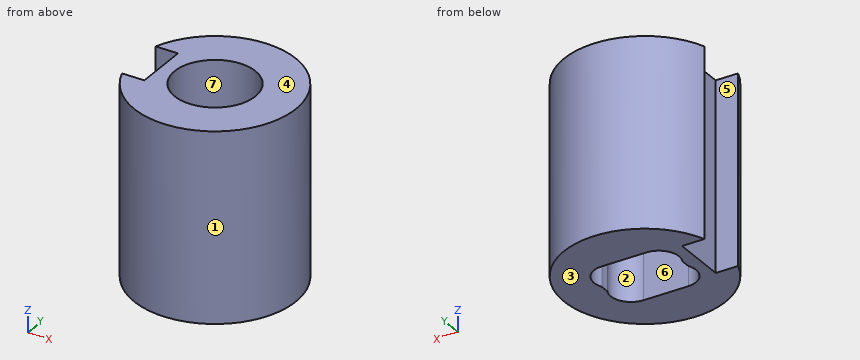
```python
from build123d import *

# Parameters (mm, degrees)
EXTRUDE_1_DEPTH     = 28
CUT_EXTRUDE_1_DEPTH = 10
SKETCH_3_R          = 6
CUT_EXTRUDE_2_DEPTH = 18


with BuildPart() as part:
    # Эскиз1 → Бобышка-Вытянуть1 (new body)
    with BuildSketch(Plane(origin=(0, 0, -1), x_dir=(-1, 0, 0), z_dir=(0, 0, -1))):
        with BuildLine():
            Line((11.313708499, 4), (8, 4))
            Line((8, 4), (8, -4))
            Line((8, -4), (11.313708499, -4))
            ThreePointArc((11.313708499, -4), (-12, 0), (11.313708499, 4))
        make_face()
    extrude(amount=-EXTRUDE_1_DEPTH)

    # Эскиз2 → Вырез-Вытянуть1 (cut)
    with BuildSketch(Plane(origin=(0, 0, -1), x_dir=(-1, 0, 0), z_dir=(0, 0, -1))):
        with BuildLine():
            Line((-3.31662479, 5), (3.31662479, 5))
            ThreePointArc((3.31662479, 5), (5.868522172, 3.577282395), (6, 0.658546503))
            Line((6, 0.658546503), (6, -0.658546503))
            ThreePointArc((6, -0.658546503), (5.868522172, -3.577282395), (3.31662479, -5))
            Line((3.31662479, -5), (-3.31662479, -5))
            ThreePointArc((-3.31662479, -5), (-5.868522172, -3.577282395), (-6, -0.658546503))
            Line((-6, -0.658546503), (-6, 0.658546503))
            ThreePointArc((-6, 0.658546503), (-5.868522172, 3.577282395), (-3.31662479, 5))
        make_face()
    extrude(amount=-CUT_EXTRUDE_1_DEPTH, mode=Mode.SUBTRACT)

    # Эскиз3 → Вырез-Вытянуть2 (cut)
    with BuildSketch(Plane.XY.offset(27)):
        Circle(SKETCH_3_R)
    extrude(amount=-CUT_EXTRUDE_2_DEPTH, mode=Mode.SUBTRACT)


solid = part.part
```
The listing builds one solid part. Answer for the finished solid, in the listing's coordinates (mm). Face numbers are marked on the shaded views. A direction names the side the tool comes from. Coordinates: 2 decimals unless noted, no trailing zeros. Loops run counter-clockwise (first coordinate to the right, second up) from the corner with the lowest first, then second, coordinate; pieces in that order, holes last. Notation, with made-up numbers: M 52.5,42 L 105.5,42 A22 ccw 105.5,69 Z; hole C 5,76 d3. An arc over 180 degrees is marked long. Answer as a JSON object with one key per item and string values. Group by question number.
Item 1: Which of the six approach directions +Z, -Z, +X, -X, +Y, -Y give full straight-line access (tool end or side, diameter ignored) to the marked faces 4, 5, 6 and 7?
Item 2: Each of these flat-tipped pins is pushed along its axis until it touches: P1, Ø1.1, axis at y = 0, z = 4, coming from the -X side; P2, Ø1, axis at y = 7.5, z = 4, coming from the -X side; P3, Ø1.5, axis at x = -5.5, y = 2, coming from the -Z side. Where does it stop, or does it pass through?
Item 3: Section B-B (z = 22) is taken. Write down the section's boundary in (x, y).
Item 4: Determine the mould class of the marked faces 1, 2 and 3 for opening direction Y: +Y half, -Y half, draft (parallel to the pull), parting line (faces both ways), or undercut.
Item 5: Consider L1, parallel to Y at x = 0, z = 16; L2, parallel to Z at x = -5.5, y = 4; L3, parallel to X at y = 1.75, z = 15.25. Determine where each line is inside the solid, lowest interval first.
Item 6: Section A-A (x = 0) is taken. Write down the section's boundary in (y, z), and give its area (3 significant figures).
Item 7: Section C-C (y = -8.75) is taken. Write down the section's boundary in (x, z).
Item 8: Section D-D (x = 9.5) is taken. Write down the section's boundary in (y, z), and give its area (3 significant figures).
Solved:
{
 "1": {"face 4": "+Z, +X, -X, +Y, -Y", "face 5": "+Z, -Z, -X", "face 6": "+Z, -Z", "face 7": "+Z"},
 "2": {"P1": "stops at x = -8", "P2": "stops at x = -9.75", "P3": "stops at z = 9"},
 "3": {"outline": "M -11.31,-4 A12 ccw long -11.31,4 L -8,4 L -8,-4 Z; hole C 0,0 d12"},
 "4": {"face 1": "parting line", "face 2": "undercut", "face 3": "draft"},
 "5": {"L1": "y = -12 to -6, 6 to 12", "L2": "z = 9 to 27", "L3": "x = -8 to -5.74, 5.74 to 11.87"},
 "6": {"outline": "M -12,-1 L -5,-1 L -5,9 L -6,9 L -6,27 L -12,27 Z; M 5,-1 L 12,-1 L 12,27 L 6,27 L 6,9 L 5,9 Z", "area": "356 mm2"},
 "7": {"outline": "M -8.21,-1 L 8.21,-1 L 8.21,27 L -8.21,27 Z"},
 "8": {"outline": "M -7.33,-1 L 7.33,-1 L 7.33,27 L -7.33,27 Z", "area": "411 mm2"}
}
